Design review of the part built by this model. Coordinates are the model's own, in mm. Face numbers are marked on the shaded views. A direction names the side the tool comes from. Coordinates: 2 decimals unless noted, no trailing zeros. Order: outer loops, then holes, each group sorted by start corner. A loop starts at its lowest first (then second) coordinate and runs counter-clockwise, first axis right, second up. Notation, with made-up numbers: (-21.5, 31.25) -> (9.5, 31.25) arc R15 cw to (9.5, 42.25) -> close; hole circle Ø10 at (-1, -17). An arc over 180 degrees is marked (long way). Use a Markdown table: item, result. Add a question column.
Q1. Wall thickness on probe 1 along X at (y, z) = (-8.25, -0.25); probe 2 along Z at (x, y) = (-2.25, 12.75); probe 3 along X at (y, z) = (-6, 2.5): over which ranges is each line inside the solid? List them lowest first.
Q2. Add section D-D (z = 16.25). State the section outline as (x, y) points.
Q3. Insertion check: pin 1 (8 mm diameter, centred on x = -6.5, z = 14.5, fed in from +Y); pin 2 (10 mm diameter, centred on y = 9, z = 7, fed in from +X); pin 3 (3 mm diameter, centred on y = -11.5, z = -2, fed in from +X). Each pin has a flat end and moves straight along its axis. Give the tip position at first contact, or say it passes through.
Q4. The part is to be moulded in two halves that separate along X. For the marked faces 3, 4 and 5, say which applies: pulls with the +X half, pulls with the -X half, needs draft (parallel to the pull), parting line crosses it, or undercut.
Q5. Add section B-B (x = 1.5). State the section outline as (y, z) points.
Q6. Add section C-C (x = -7). State the section outline as (y, z) points, then the cut area to 3 significant figures.
Q7. Machinability: for the marked faces 1 and 2, which of the approach directions +Z, -Z, +X, -X, +Y, -Y give a long, thin tool a straight path to every point of the face, cutting with its end or side? Answer none if there is none.
Q8. Add section A-A (y = 0). State the section outline as (x, z) points.
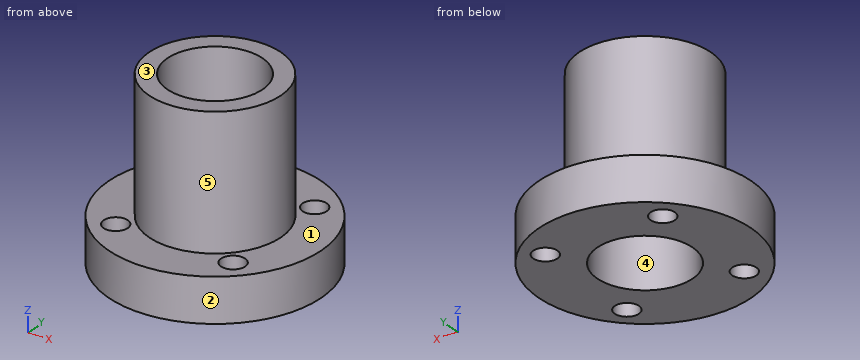
from build123d import *

# Parameters (mm, degrees)
F0_R     = 14.5
F0_R_2   = 9
F1_DEPTH = 6
F2_DEPTH = 18
F4_D     = 13
F6_D     = 3.3


with BuildPart() as f1:
    # F0 (on Top) → F1 (new body)
    with BuildSketch(Plane.XY):
        Circle(F0_R)
        Circle(F0_R_2, mode=Mode.SUBTRACT)
        Circle(F0_R_2)
    extrude(amount=-F1_DEPTH)

    # F0 (on Top) → F2 (join)
    with BuildSketch(Plane.XY):
        Circle(F0_R_2)
    extrude(amount=F2_DEPTH)

    # F4 (through all)
    with Locations(Plane.XY.offset(18)):
        with Locations((0, 0)):
            Hole(F4_D / 2)

    # F6 (through all)
    with Locations(Plane(origin=(0, 0, -6), x_dir=(1, 0, 0), z_dir=(0, 0, -1))):
        with Locations((8.0136820347, 7.9841035315), (8.0136820347, -8.0158964685), (-7.9863179653, -8.0158964685), (-7.9863179653, 7.9841035315)):
            Hole(F6_D / 2)


solid = f1.part
Established:
| question | item | result |
|---|---|---|
| 1 | probe 1 | -11.92 to -9.61, -6.36 to 6.39, 9.64 to 11.92 |
| 1 | probe 2 | -6 to 0 |
| 1 | probe 3 | -6.71 to -2.5, 2.5 to 6.71 |
| 2 | outline | circle Ø18 at (0, 0); hole circle Ø13 at (0, 0) |
| 3 | pin 1 | y = 8.65 |
| 3 | pin 2 | x = 8.06 |
| 3 | pin 3 | x = 10.5 |
| 4 | face 3 | needs draft |
| 4 | face 4 | undercut |
| 4 | face 5 | parting line crosses it |
| 5 | outline | (-14.42, -6) -> (-6.32, -6) -> (-6.32, 18) -> (-8.87, 18) -> (-8.87, 0) -> (-14.42, 0) -> close; (6.32, -6) -> (14.42, -6) -> (14.42, 0) -> (8.87, 0) -> (8.87, 18) -> (6.32, 18) -> close |
| 6 | outline | (-12.7, -6) -> (-9.31, -6) -> (-9.31, 0) -> (-12.7, 0) -> close; (-6.66, -6) -> (6.69, -6) -> (6.69, 0) -> (5.66, 0) -> (5.66, 18) -> (-5.66, 18) -> (-5.66, 0) -> (-6.66, 0) -> close; (9.34, -6) -> (12.7, -6) -> (12.7, 0) -> (9.34, 0) -> close |
| 6 | area | 324 mm^2 |
| 7 | face 1 | +Z |
| 7 | face 2 | +Z, -Z |
| 8 | outline | (-14.5, -6) -> (-6.5, -6) -> (-6.5, 18) -> (-9, 18) -> (-9, 0) -> (-14.5, 0) -> close; (6.5, -6) -> (14.5, -6) -> (14.5, 0) -> (9, 0) -> (9, 18) -> (6.5, 18) -> close |
